Part model, mm, in its own coordinate system. Give positions to 0.01 mm unless a question says otherwise; leave off trailing zeros. Write each loop counter-clockwise with the first axis right and the second up, starting at its lowest first coordinate (ties: lowest second). Pieces come first, ordered by that corner, then holes.
from build123d import *

# Parameters (mm, degrees)
SKETCH1_W           = 88.9
SKETCH1_H           = 76.2
BOSS_EXTRUDE1_DEPTH = 1.6
SKETCH2_R           = 1.5875
CUT_EXTRUDE1_DEPTH  = 2.6
SKETCH4_R           = 1.905
CUT_EXTRUDE2_DEPTH  = 2.6
FILLET1_R           = 6.35


with BuildPart() as part:
    # Sketch1 → Boss-Extrude1 (new body)
    with BuildSketch(Plane.XY):
        with Locations((28.959521177, 30.063142475)):
            Rectangle(SKETCH1_W, SKETCH1_H)
    extrude(amount=BOSS_EXTRUDE1_DEPTH)

    # Sketch2 → Cut-Extrude1 (cut, through all)
    with BuildSketch(Plane(origin=(0, 0, 0), x_dir=(-1, 0, 0), z_dir=(0, 0, -1))):
        with Locations((5.140478823, 57.813142475)):
            Circle(SKETCH2_R)
        with Locations((-21.859521177, 57.813142475)):
            Circle(SKETCH2_R)
        with Locations((-21.859521177, 40.813142475)):
            Circle(SKETCH2_R)
        with Locations((5.140478823, 40.813142475)):
            Circle(SKETCH2_R)
    extrude(amount=-CUT_EXTRUDE1_DEPTH, mode=Mode.SUBTRACT)

    # Sketch4 → Cut-Extrude2 (cut, through all)
    with BuildSketch(Plane(origin=(0, 0, 0), x_dir=(-1, 0, 0), z_dir=(0, 0, -1))):
        with Locations((10.410478823, 63.083142475)):
            Circle(SKETCH4_R)
        with Locations((-68.329521177, 63.083142475)):
            Circle(SKETCH4_R)
        with Locations((-68.329521177, -2.956857525)):
            Circle(SKETCH4_R)
        with Locations((10.410478823, -2.956857525)):
            Circle(SKETCH4_R)
    extrude(amount=-CUT_EXTRUDE2_DEPTH, mode=Mode.SUBTRACT)

    # Fillet1
    fillet1_edges = [part.edges().sort_by_distance(p)[0] for p in [
        (-15.490478823, 68.163142475, 0.8),
        (73.409521177, 68.163142475, 0.8),
        (73.409521177, -8.036857525, 0.8),
        (-15.490478823, -8.036857525, 0.8),
    ]]
    fillet(fillet1_edges, radius=FILLET1_R)


solid = part.part
1) Drill centre lines: L1, parallel to X at y = 58, z = 0.3; L2, parallel to Y at x = -5.5, z = 1; L3, parallel to X at y = 42, z = 0.3. Where is each one in solid material? Low to high.
Check result:
L1: x = -15.49 to -6.72, -3.56 to 20.28, 23.44 to 73.41
L2: y = -8.04 to 39.27, 42.36 to 56.27, 59.36 to 68.16
L3: x = -15.49 to -6.19, -4.09 to 20.81, 22.91 to 73.41
2) Saw through at A-A (x = 22). Write the cut outline in (y, z), and give its area (3 significant figures).
Check result:
outline: (-8.04, 0) - (39.23, 0) - (39.23, 1.6) - (-8.04, 1.6) - close; (42.39, 0) - (56.23, 0) - (56.23, 1.6) - (42.39, 1.6) - close; (59.39, 0) - (68.16, 0) - (68.16, 1.6) - (59.39, 1.6) - close
area: 112 mm2
3) Flat gauge pin, fed straight in: P1, Ø2.5, axis at x = 68.33, y = 63.08, coming from the +Z side. Where does the tip first touch, or does it go through?
Check result:
P1: passes through
4) Mould opens along Y. For faces 1 (the cylindrical face through (71.5, -6.226, 0.811)), 2 (the flat face through (28, 31, 1.6)), 3 (the cylindrical face through (-4.934, 59.387, 0.789)) say: +Y half, -Y half, draft (parallel to the pull), parting line (faces both ways), or undercut.
Check result:
face 1: -Y half
face 2: draft
face 3: undercut
5) Saw through at B-B (z = 0.6). State how many separate pieces and enclosed holes the cut face has, and give its area (3 significant figures).
Check result:
separate pieces: 1
enclosed holes: 8
area: 6,660 mm2
